Input: dimensioned drawing with shaded views. Units: mm. Origin: part minimum x, y, z. A direction names the side the tool comes from. Give positions to 0.01 mm unless a question says otherwise; leave off trailing zeros. Order: outer loops, then holes, each group sorted by start corner. A loop starts at its lowest first (then second) coordinate and runs counter-clockwise, first axis right, second up. Notation, with made-up numbers: M -4,34.25 L 41,34.25 A21 ccw 41,45.25 Z; hole C -27.75,80.25 d5. An arc over 180 degrees is marked long. Answer in a Markdown table with one row per item. Add a question column.
(1) Set-up query: the marked faces 1, 2 and 3. Return all of +Z, -Z, +X, -X, +Y, -Y with unobstructed straight access to the full face (end or side cutting, diameter ignored); none if empty.
(2) Section query A-A, the plane z = 27. Return loops of the section in (x, y), plus the area to 3 significant figures.
(3) Section query D-D, the plane y = 6.5. Return loops of the section in (x, z).
(4) Material intervals for line 1 along X through (y, z) = (15, 46); line 2 along Y through (x, z) = (7, 10); line 3 along Z through (x, y) = (42.5, 38), sorted ascending.
(5) Mould query, pull axis X, two halves, no side actions, for the marked faces 4, 5, 6 and 7. Classes: pulls with the +X half, pulls with the -X half, needs draft (parallel to the pull), parting line crosses it, or undercut.
(6) Pin query (flat end, axial travel): P1, Ø9, axis at y = 15, z = 45.5, coming from the -X side; P2, Ø4, axis at x = 45, y = 21, coming from the -Z side; P3, Ø4, axis at y = 38.5, z = 19.5, coming from the -X side. Return the tip coordinate at first contact, or that it passes through.
(7) Section query B-B, the plane x = 25. Return loops of the section in (y, z), plus the area to 3 significant figures.
(8) Section query C-C, the plane y = 17.5. Return loops of the section in (x, z), plus the area to 3 significant figures.
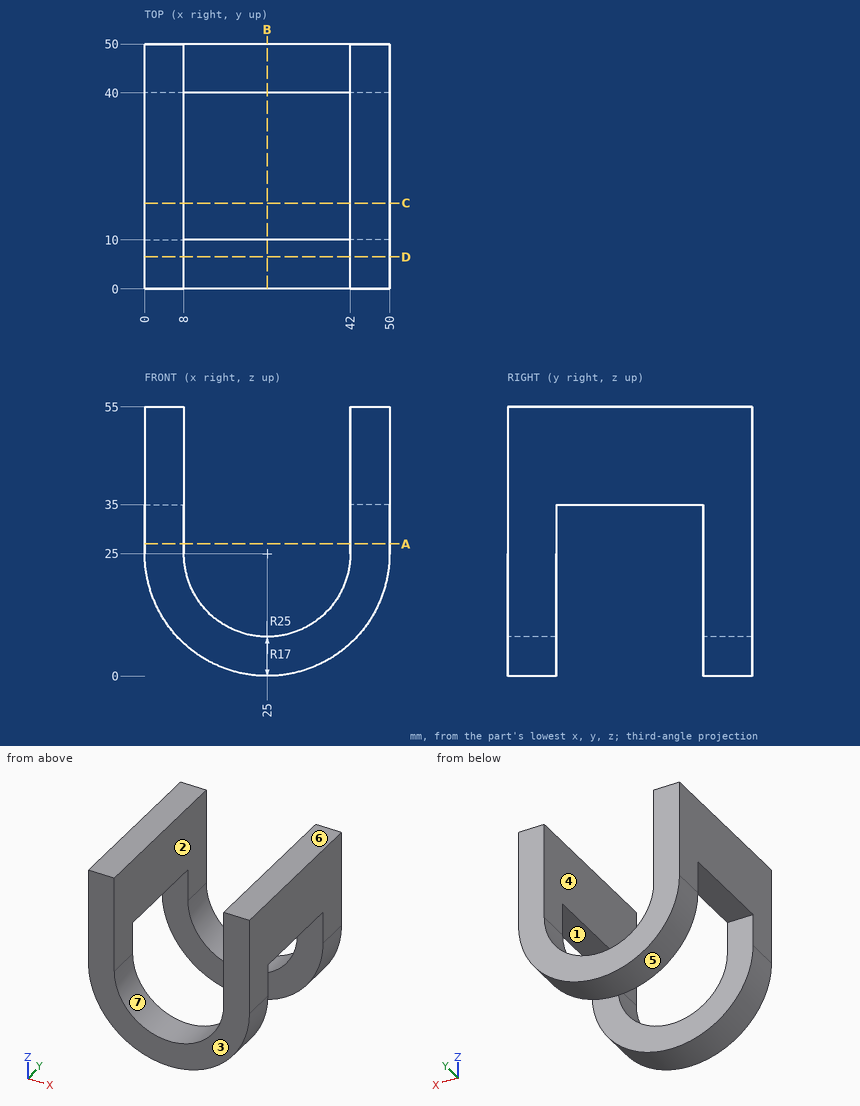
Values follow:
| question | item | result |
|---|---|---|
| 1 | face 1 | -Z, +X, -X |
| 1 | face 2 | +Z, +Y, -Y |
| 1 | face 3 | +Z, -Z, +X, -X, -Y |
| 2 | outline | M 0,0 L 8,0 L 8,10 L 0,10 Z; M 0,40 L 8,40 L 8,50 L 0,50 Z; M 42,0 L 50,0 L 50,10 L 42,10 Z; M 42,40 L 50,40 L 50,50 L 42,50 Z |
| 2 | area | 320 mm² |
| 3 | outline | M 0,25 A25 ccw 50,25 L 50,55 L 42,55 L 42,25 A17 cw 8,25 L 8,55 L 0,55 Z |
| 4 | line 1 | x = 0 to 8, 42 to 50 |
| 4 | line 2 | y = 0 to 10, 40 to 50 |
| 4 | line 3 | z = 35 to 55 |
| 5 | face 4 | undercut |
| 5 | face 5 | parting line crosses it |
| 5 | face 6 | needs draft |
| 5 | face 7 | undercut |
| 6 | P1 | stops at x = 0 |
| 6 | P2 | stops at z = 35 |
| 6 | P3 | stops at x = 0.35 |
| 7 | outline | M 0,0 L 10,0 L 10,8 L 0,8 Z; M 40,0 L 50,0 L 50,8 L 40,8 Z |
| 7 | area | 160 mm² |
| 8 | outline | M 0,35 L 8,35 L 8,55 L 0,55 Z; M 42,35 L 50,35 L 50,55 L 42,55 Z |
| 8 | area | 320 mm² |
